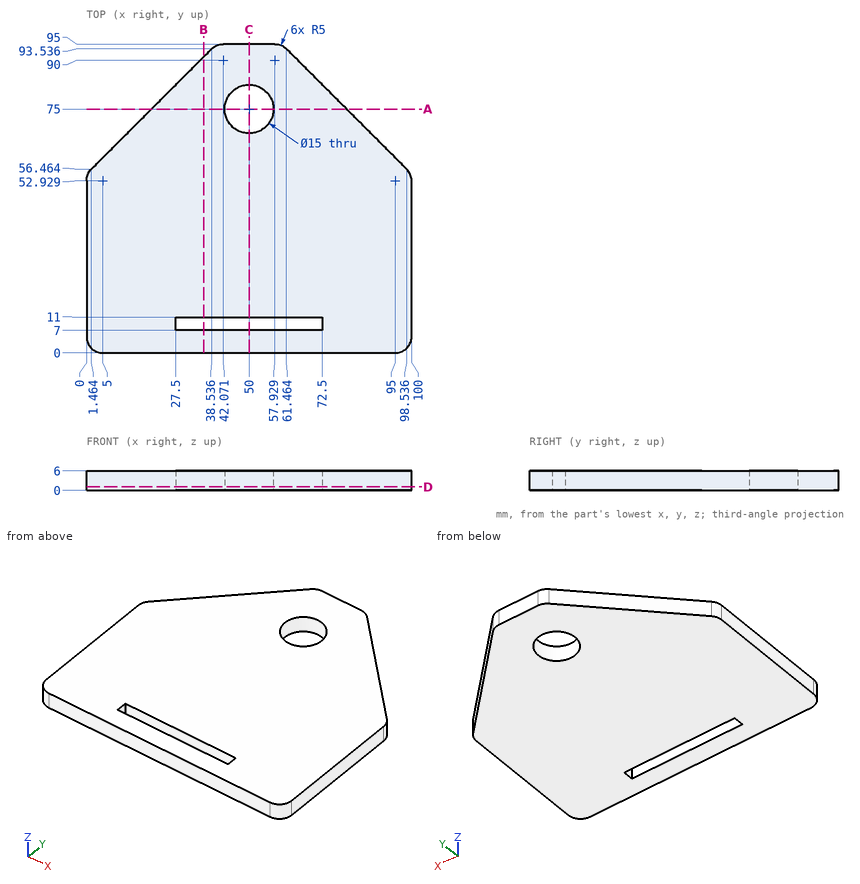
Design review of the part shown in the three views and the two pictorial views. Dimensions are in mm from the part's minimum x, y and z. Round coordinates to 2 decimals unless told otherwise and drop trailing zeros. Order: outer loops, then holes, each group sorted by start corner. A loop starts at its lowest first (then second) coordinate and runs counter-clockwise, first axis right, second up.
Item 1: Add section C-C, the plane x = 50. State the section outline as (y, z) points.
Working result:
outline: (0, 0) - (7, 0) - (7, 6) - (0, 6) - close; (11, 0) - (67.5, 0) - (67.5, 6) - (11, 6) - close; (82.5, 0) - (95, 0) - (95, 6) - (82.5, 6) - close
Item 2: For pin 1 (3 mm diameter, centred on x = 85.5, y = 57, fed in from -Z); pin 2 (9 mm diameter, centred on x = 50, y = 75, fed in from -Z); pin 3 (3 mm diameter, centred on y = 55.5, z = 4, fed in from +X); pin 4 (1.8 mm diameter, centred on x = 59.5, z = 4, fed in from +Y) (1 decimal), all flat-tipped, find the tip position at first contact; note any pin that passes through.
Working result:
pin 1: stops at z = 0
pin 2: passes through
pin 3: stops at x = 99.88
pin 4: stops at y = 95
Item 3: Add section D-D, the plane z = 1.05. State the section outline as (x, y) points (1 decimal), and give its area (3 significant figures).
Working result:
outline: (0, 5) arc R5 ccw to (5, 0) - (95, 0) arc R5 ccw to (100, 5) - (100, 52.9) arc R5 ccw to (98.5, 56.5) - (61.5, 93.5) arc R5 ccw to (57.9, 95) - (42.1, 95) arc R5 ccw to (38.5, 93.5) - (1.5, 56.5) arc R5 ccw to (0, 52.9) - close; hole (27.5, 7) - (72.5, 7) - (72.5, 11) - (27.5, 11) - close; hole circle Ø15 at (50, 75)
area: 7,530 mm2
Item 4: To check wall thickness, follow probe 1 along Y at (x, z) = (50, 2.4); probe 2 along Y at (x, z) = (45, 0.65); probe 3 along X at (y, z) = (75, 4.6). State the ranges of each line that lie inside material, in increasing order.
Working result:
probe 1: y = 0 to 7, 11 to 67.5, 82.5 to 95
probe 2: y = 0 to 7, 11 to 69.41, 80.59 to 95
probe 3: x = 20 to 42.5, 57.5 to 80
Item 5: Add section A-A, the plane y = 75. State the section outline as (x, z) points, and give its area (3 significant figures).
Working result:
outline: (20, 0) - (42.5, 0) - (42.5, 6) - (20, 6) - close; (57.5, 0) - (80, 0) - (80, 6) - (57.5, 6) - close
area: 270 mm2
Item 6: Add section B-B, the plane x = 36. State the section outline as (y, z) points, and give its area (3 significant figures).
Working result:
outline: (0, 0) - (7, 0) - (7, 6) - (0, 6) - close; (11, 0) - (91, 0) - (91, 6) - (11, 6) - close
area: 522 mm2
